Autodesk Inventor part; units mm, degrees
ref_plane "YZ Plane" through (0, 0, 0) normal (1, 0, 0) x (0, 1, 0)
ref_plane "XZ Plane" through (0, 0, 0) normal (0, 1, 0) x (-1, 0, 0)
ref_plane "XY Plane" through (0, 0, 0) normal (0, 0, 1) x (1, 0, 0)
sketch "Sketch1" plane through (0, 0, 0) normal (0, 1, 0) x (-1, 0, 0)
  circle A0 centre (0, 0) radius 11
  dimension "d0" = 22
extrude "Extrusion1" add sketch "Sketch1" along normal blind 8.5
sketch "Sketch2" plane through (0, 8.5, 0) normal (0, 1, 0) x (1, 0, 0)
  circle A0 centre (0, 0) radius 2.5
  dimension "d3" = 5
extrude "Extrusion2" add sketch "Sketch2" along normal blind 2.6
chamfer "Chamfer1" distance 1.5 angle 30 1 edges at (11, 8.5, 0) measured on face at (-8.0601, 8.5, -0.8775)
sketch "Sketch3" plane through (0, 0, 0) normal (0, -1, 0) x (1, 0, 0)
  circle A0 centre (0, 0) radius 10.25
  dimension "d9" = 20.5
extrude "Extrusion3" cut sketch "Sketch3" against normal blind 7
sketch "Sketch4" plane through (0, 8.5, 0) normal (0, 1, 0) x (1, 0, 0)
  circle A0 centre (0, 0) radius 2.5
  circle A1 centre (0, 0) radius 9.5
  line L0 (-2.9, 5.1) -> (2.9, 5.1)
  line L1 (2.9, 5.1) -> (2.9, -5.1)
  line L2 (2.9, -5.1) -> (-2.9, -5.1)
  line L3 (-2.9, -5.1) -> (-2.9, 5.1)
  line L4 (-2.9, 5.1) -> (2.9, -5.1) construction
  line L5 (2.9, 5.1) -> (-2.9, -5.1) construction
  dimension "d12" = 5.8
  dimension "d13" = 10.2
hole "Hole1" at (-2.9, 8.5, -5.1) at (2.9, 8.5, -5.1) at (-2.9, 8.5, 5.1) at (2.9, 8.5, 5.1) direction (0, -1, 0) diameter 1.6 depth 17
sketch "Sketch5" plane through (0, 0, 0) normal (0, -1, 0) x (1, 0, 0)
  circle A0 centre (-2.9, 5.1) radius 0.8
  circle A1 centre (-2.9, -5.1) radius 0.8
  circle A2 centre (2.9, -5.1) radius 0.8
  circle A3 centre (2.9, 5.1) radius 0.8
  circle A4 centre (0, 0) radius 10.25
  circle A5 centre (0, 0) radius 10.25
  circle A6 centre (0, 0) radius 11
  line L0 (-10.5, -1.4) -> (-10, -1.4)
  line L1 (-10, -1.4) -> (-10, 1.4)
  line L2 (-10, 1.4) -> (-10.5, 1.4)
  line L3 (-10.5, 1.4) -> (-10.5, -1.4)
  line L4 (-10.5, -1.4) -> (-10, 1.4) construction
  line L5 (-10, -1.4) -> (-10.5, 1.4) construction
  line L6 (0, 0) -> (-10.25, 0)
  dimension "d21" = 0.5
  dimension "d22" = 2.8
extrude "Extrusion4" add sketch "Sketch5" against normal blind 7 contours L2 L1 L6 A4 | A4 L0 L3 L2 | A4 L6 L1 L0
pattern_circular "Circular Pattern1" count 18 over 360 about axis through (0, 0, 0) along (0, 1, 0) of "Extrusion4"
properties part number "burshless_20_top"
CAD build for the part. Positions are in the model's coordinates, mm. A direction names the side the tool comes from. Coordinates: 2 decimals unless noted, no trailing zeros. Write each loop counter-clockwise with the first axis right and the second up, starting at its lowest first coordinate (ties: lowest second). Pieces come first, ordered by that corner, then holes. Notation, with made-up numbers: (3, 88.25) -> (22, 88.25) arc R27 cw to (22, 109.25) -> close; hole circle Ø4 at (41, 66). An arc over 180 degrees is marked (long way). Return JSON: item names as keys, results as strings. Group by question number.
Q1. Which spindle directions (+Z, -Z, +X, -X, +Y, -Y) get a long thin tool onto all of the face, cutting with end or side? Do faces 5 (the face through (-9.404, 3.451, 3.402)), 6 (the face through (2.107, 7.74, -5.204)), 7 (the face through (-2, 8.5, -2)). Say none if no direction does.
Q2. Cut at B-B, the plane z = 0. Give the cut face in (x, y), then the cut area to 3 significant figures.
Q3. Cut at A-A, the plane x = 0. Give the cut face in (y, z), then the cut area to 3 significant figures.
Q4. Flat gauge pins, fed straight in: pin 1 (6 mm diameter, centred on x = -5, z = -8, fed in from +Y); pin 2 (4 mm diameter, centred on x = 0.5, z = 6, fed in from -Y); pin 3 (6 mm diameter, centred on x = -4.5, y = 6.5, fed in from -Z). Where does each tip first touch, or does it go through?
Q5. Cut at C-C, the plane y = 8. Give the cut face in (x, z), then the cut area to 3 significant figures.
Q6. Drill centre lines: line 1 (Z direction, x = -2.9, y = 7.45); line 2 (Z direction, x = -2.9, y = 8.1); line 3 (Y direction, x = -2.75, z = 6). Where is each one in solid material? Low to high.
Q7. Pull direction Z, two halves, no side cores. Call faces 1 (the face through (-0.54, 9.78, -2.44)), 2 (the face through (7.673, 3.451, -6.413)), 3 (the face through (2, 0, -10)), 4 (the face through (10, 3, 0)): released by +Z, released by -Z, zero draft, split by the parting line, or undercut.
Returned:
{
 "1": {"face 5": "-Y", "face 6": "+Y, -Y", "face 7": "+Y"},
 "2": {"outline": "(-11, 0) -> (-10, 0) -> (-10, 7) -> (10, 7) -> (10, 0) -> (11, 0) -> (11, 7.63) -> (9.5, 8.5) -> (2.5, 8.5) -> (2.5, 11.1) -> (-2.5, 11.1) -> (-2.5, 8.5) -> (-9.5, 8.5) -> (-11, 7.63) -> close", "area": "58.7 mm2"},
 "3": {"outline": "(0, -11) -> (7.63, -11) -> (8.5, -9.5) -> (8.5, -2.5) -> (11.1, -2.5) -> (11.1, 2.5) -> (8.5, 2.5) -> (8.5, 9.5) -> (7.63, 11) -> (0, 11) -> (0, 10.25) -> (7, 10.25) -> (7, -10.25) -> (0, -10.25) -> close", "area": "55.2 mm2"},
 "4": {"pin 1": "stops at y = 8.5", "pin 2": "stops at y = 7", "pin 3": "stops at z = -10.9"},
 "5": {"outline": "circle Ø20.73 at (0, 0); hole circle Ø1.6 at (-2.9, -5.1); hole circle Ø1.6 at (-2.9, 5.1); hole circle Ø1.6 at (2.9, -5.1); hole circle Ø1.6 at (2.9, 5.1)", "area": "330 mm2"},
 "6": {"line 1": "z = -10.61 to -5.9, -4.3 to 4.3, 5.9 to 10.61", "line 2": "z = -9.77 to -5.9, -4.3 to 4.3, 5.9 to 9.77", "line 3": "y = 7 to 8.5"},
 "7": {"face 1": "split by the parting line", "face 2": "undercut", "face 3": "zero draft", "face 4": "undercut"}
}
